```python
from build123d import *

# Parameters (mm, degrees)
F1_DEPTH = 1.5
F2_R     = 1.49999
F3_R     = 7
F4_DEPTH = 3
F5_R     = 4
F6_DEPTH = 25


# Not quite as in the source:
# - a fillet or chamfer is up to 0.001 mm smaller than in the source, because OpenCascade refuses the exact size


with BuildPart() as f1:
    # F0 (on Front) → F1 (new body, symmetric)
    with BuildSketch(Plane.XZ):
        with BuildLine():
            ThreePointArc((-11.990991839, 5.0892857143), (-20.2324383609, 6.9845386823), (-25, 0))
            Line((-25, 0), (-25, -2))
            Line((-25, -2), (-22, -2))
            Line((-22, -2), (-22, 0))
            ThreePointArc((-22, 0), (-19.1394630165, 4.1907232094), (-14.1945951034, 3.0535714286))
            ThreePointArc((-14.1945951034, 3.0535714286), (-11.0249907967, 0.7968088775), (-7.2165180994, 0))
            Line((-7.2165180994, 0), (0, 0))
            Line((0, 0), (7.2165180994, 0))
            ThreePointArc((7.2165180994, 0), (11.0249907967, 0.7968088775), (14.1945951034, 3.0535714286))
            ThreePointArc((14.1945951034, 3.0535714286), (19.1394630165, 4.1907232094), (22, 0))
            Line((22, 0), (22, -2))
            Line((22, -2), (25, -2))
            Line((25, -2), (25, 0))
            ThreePointArc((25, 0), (20.2324383609, 6.9845386823), (11.990991839, 5.0892857143))
            ThreePointArc((11.990991839, 5.0892857143), (9.822315208, 3.5451850215), (7.2165180994, 3))
            Line((7.2165180994, 3), (0, 3))
            Line((0, 3), (-7.2165180994, 3))
            ThreePointArc((-7.2165180994, 3), (-9.822315208, 3.5451850215), (-11.990991839, 5.0892857143))
        make_face()
    extrude(amount=F1_DEPTH, both=True)

    # F2 (radius 1.5 in the source; OpenCascade refuses exactly that, so slightly less here)
    f2_edges = [f1.edges().sort_by_distance(p)[0] for p in [
        (-20.232438, -1.5, 6.984539),
        (-19.139463, -1.5, 4.190723),
        (-20.232438, 1.5, 6.984539),
        (-19.139463, 1.5, 4.190723),
    ]]
    fillet(f2_edges, radius=F2_R)

    # F3 (on Top) → F4 (join)
    with BuildSketch(Plane.XY):
        Circle(F3_R)
    extrude(amount=F4_DEPTH)

    # F5 (on face) → F6 (cut)
    with BuildSketch(Plane.XY.offset(3)):
        Circle(F5_R)
    extrude(amount=-F6_DEPTH, mode=Mode.SUBTRACT)


solid = f1.part
```
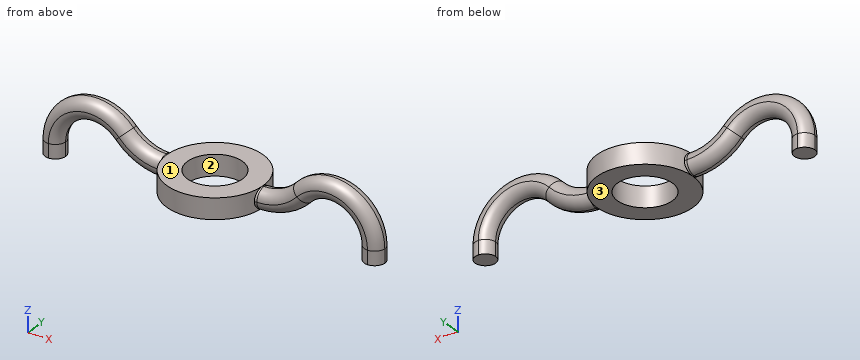
Input: part model. Units: mm. Frame: model coordinates. Face numbers are marked on the shaded views. A direction names the side the tool comes from. Give positions to 0.01 mm unless a question says otherwise; leave off trailing zeros. Loops run counter-clockwise (first coordinate to the right, second up) from the corner with the lowest first, then second, coordinate; pieces in that order, holes last. Notation, with made-up numbers: M 39.25,10 L 70.25,10 A20 cw 70.25,46 Z; hole C -7,40 d10. An arc over 180 degrees is marked long. Answer as CSV lines item,"result". Start each with the question number.
1. Reachability of the marked faces 1, 2 and 3 from +Z, -Z, +X, -X, +Y, -Y: full face, straight path, thin tool, end or side. Return the list, or none.
2. Line query: L1, parallel to X at y = -0.5, z = 2; L2, parallel to X at y = -0.25, z = 1.75; L3, parallel to X at y = 1.25, z = -1.5. Output: solid intervals per line, ascending.
3. Section B-B on y = -2.5. Return loops of the section in (x, z).
4. Pin query (flat end, axial travel): P1, Ø4, axis at x = 2.5, y = 2.5, coming from the +Z side; P2, Ø1.5, axis at x = -6, z = 3.5, coming from the +Y side; P3, Ø8, axis at x = -9, y = 4.5, coming from the +Z side. Return the tip coordinate at first contact, or that it passes through.
5. Section D-D on y = -5.5. Return loops of the section in (x, z), plus the area to 3 significant figures.
6. Section C-C on z = 1. State how many separate pieces and enclosed holes the cut face has, plus the area to 3 significant figures.
7. Section A-A on x = 0. Return loops of the section in (y, z).
Computed values:
1,face 1,"+Z, +Y, -Y"
1,face 2,"+Z, -Z"
1,face 3,"-Z, +Y, -Y"
2,L1,"x = -24.64 to -21.63, -12.91 to -3.97, 3.97 to 12.91, 21.63 to 24.64"
2,L2,"x = -24.77 to -21.67, -12.67 to -3.99, 3.99 to 12.67, 21.67 to 24.77"
2,L3,"x = -24.33 to -22.67, 22.67 to 24.33"
3,outline,"M -6.54,0 L -3.12,0 L -3.12,3 L -6.54,3 Z; M 3.12,0 L 6.54,0 L 6.54,3 L 3.12,3 Z"
4,P1,"stops at z = 3"
4,P2,"stops at y = 4.4"
4,P3,"stops at z = 3.71"
5,outline,"M -4.33,0 L 4.33,0 L 4.33,3 L -4.33,3 Z"
5,area,"26.0 mm²"
6,separate pieces,"3"
6,enclosed holes,"1"
6,area,"139 mm²"
7,outline,"M -7,0 L -4,0 L -4,3 L -7,3 Z; M 4,0 L 7,0 L 7,3 L 4,3 Z"
